Geometry check sheet. Reference: the model listing, model coordinates, mm. A direction names the side the tool comes from. Coordinates: 2 decimals unless noted, no trailing zeros. Loops run counter-clockwise (first coordinate to the right, second up) from the corner with the lowest first, then second, coordinate; pieces in that order, holes last. Notation, with made-up numbers: (58, 34) - (74, 34) arc R25 cw to (74, 70) - close; hole circle Ø2 at (31.25, 81). An arc over 180 degrees is marked (long way). Write item = value, one per line. Start each with the question number.
from build123d import *

# Parameters (mm, degrees)
SKETCH2_W           = 20
SKETCH2_H           = 50
BOSS_EXTRUDE1_DEPTH = 3
SKETCH3_W           = 3
SKETCH3_H           = 20
BOSS_EXTRUDE2_DEPTH = 20
SKETCH4_W           = 20
SKETCH4_H           = 3
BOSS_EXTRUDE3_DEPTH = 84


with BuildPart() as part:
    # Sketch2 → Boss-Extrude1 (new body)
    with BuildSketch(Plane(origin=(23.311118251, -39.089251492, 0), x_dir=(0, 0, 1), z_dir=(-0.5121927738543929, 0.8588705155093768, 0))):
        with Locations((18.034703764, 62.678269869)):
            Rectangle(SKETCH2_W, SKETCH2_H)
    extrude(amount=BOSS_EXTRUDE1_DEPTH)

    # Sketch3 → Boss-Extrude2 (add)
    with BuildSketch(Plane.XY.offset(28.034703764)):
        with Locations((97.115399092, 15.818924759)):
            Rectangle(SKETCH3_W, SKETCH3_H)
    extrude(amount=-BOSS_EXTRUDE2_DEPTH)

    # Sketch4 → Boss-Extrude3 (add)
    with BuildSketch(Plane.ZY.offset(-95.615399092)):
        with Locations((18.034703764, 24.318924759)):
            Rectangle(SKETCH4_W, SKETCH4_H)
    extrude(amount=BOSS_EXTRUDE3_DEPTH)


solid = part.part
(1) Tool access check on faces 4 (the face through (65, 23, 8.035)), 5 (the face through (75.17, -4.67, 17.89)). Record the directions out of +Z, -Z, +X, -X, +Y, -Y that give a thin tool (end or side, any length) a straight path to the whole face; none if there is none.
(2) Scan lines: line 1 (Y direction, x = 36, z = 26.5); line 2 (Y direction, x = 95.5, z = 15); line 3 (Y direction, x = 85.5, z = 19.75). Record each from-to range of solid material in increasing order.
(3) Sectioned sample at C-C on y = 14.5. Enter the section's corners in (x, z).
(4) Sectioned sample at B-B on x = 59. Enter the section's corners in (y, z).
(5) Sectioned sample at D-D on x = 34.5. Enter the section's corners in (y, z).
(6) Draft check along Y on faces 1 (the face through (11.615, 24, 18)), 2 (the face through (54.9, -18.5, 17.9)), 3 (the face through (54, 22.819, 18)). Enter one of: pulls with the +Y half, pulls with the -Y half, needs draft (parallel to the pull), parting line crosses it, or undercut.
(7) Sectioned sample at A-A on z = 26.5. Enter the section's corners in (x, y), plus the area to 3 significant figures.
(8) Depth check by flat-ended pin: pin 1 (8 mm diameter, centred on x = 26, z = 21.5, fed in from -Y); pin 2 (3 mm diameter, centred on y = -7, z = 12.5, fed in from -X); pin 3 (4 mm diameter, centred on x = 66, z = 23.5, fed in from -Y). Enter the tip coordinate at first touch or a pass-through.
Working result:
q1.face_4 = -Z, +X, -X, +Y, -Y
q1.face_5 = +Z, -Z, -X
q2.line_1 = 22.82 to 25.82
q2.line_2 = 3.96 to 7.45, 22.82 to 25.82
q2.line_3 = -2 to 1.49, 22.82 to 25.82
q3.outline = (95.62, 8.03) - (98.62, 8.03) - (98.62, 28.03) - (95.62, 28.03) - close
q4.outline = (-17.81, 8.03) - (-14.31, 8.03) - (-14.31, 28.03) - (-17.81, 28.03) - close; (22.82, 8.03) - (25.82, 8.03) - (25.82, 28.03) - (22.82, 28.03) - close
q5.outline = (22.82, 8.03) - (25.82, 8.03) - (25.82, 28.03) - (22.82, 28.03) - close
q6.face_1 = needs draft
q6.face_2 = pulls with the -Y half
q6.face_3 = undercut
q7.outline = (11.62, 22.82) - (95.62, 22.82) - (95.62, 7.52) - (54.14, -17.21) - (55.67, -19.79) - (98.62, 5.82) - (98.62, 25.82) - (11.62, 25.82) - close
q7.area = 457 mm2
q8.pin_1 = 22.82
q8.pin_2 = 68.75
q8.pin_3 = -14.82
